Can you work these out from the model? Positions are in its coordinate system, mm. A direction names the side the tool comes from. Give positions to 0.01 mm unless a question says otherwise; leave off trailing zeros. Loops run counter-clockwise (first coordinate to the right, second up) from the corner with the lowest first, then second, coordinate; pieces in that order, holes last. Notation, with made-up numbers: (54, -3) - (93, -3) arc R10 cw to (93, 11) - close; hole circle Ø2 at (76.25, 87). An arc over 180 degrees is marked (long way). Answer as a JSON object with one key per item and string values.
```python
from build123d import *

# Parameters (mm, degrees)
F1_DEPTH = 100
F2_W     = 150
F2_H     = 99.866986
F3_DEPTH = 20
F4_R     = 5
F5_DEPTH = 15


with BuildPart() as f1:
    # F0 (on Top) → F1 (new body)
    with BuildSketch(Plane.XY):
        Polygon((-75, -10), (75, -10), (-75, 10), align=None)
    extrude(amount=F1_DEPTH)

    # F2 (on face) → F3 (join)
    with BuildSketch(Plane.XZ.offset(10)):
        with Locations((0, 49.933493)):
            Rectangle(F2_W, F2_H)
    extrude(amount=F3_DEPTH)

    # F4 (on face) → F5 (join)
    with BuildSketch(Plane(origin=(0, 0, 0), x_dir=(-0.991228, 0.132164, 0), z_dir=(0.132164, 0.991228, 0))):
        with Locations((-68.66373, 45)):
            Circle(F4_R)
    extrude(amount=F5_DEPTH)


solid = f1.part
```
1) I'm going to push a flat-ended pin straight in: P1, Ø2, axis at x = 43.5, y = -21, coming from the +Z side. Where does the tip first touch, or does it pass through?
Check sheet entries:
{"P1": "z = 99.87"}
2) Imagine slicing it at C-C on x = -2.5. Write out the boundary of the cut face in (y, z).
Check sheet entries:
{"outline": "(-30, 0) - (0.33, 0) - (0.33, 100) - (-10, 100) - (-10, 99.87) - (-30, 99.87) - close"}
3) I need wall thicknesses on L1, parallel to Z at x = 1, y = -16.5; L2, parallel to Y at x = 0, z = 16; L3, parallel to Y at x = -7.5, z = 10.5. Which ranges of each line are inside material? Lowest first, please.
Check sheet entries:
{"L1": "0 to 99.87", "L2": "-30 to 0", "L3": "-30 to 1"}
4) Imagine slicing it at A-A on x = -48. Write out the boundary of the cut face in (y, z), and give its area (3 significant figures).
Check sheet entries:
{"outline": "(-30, 0) - (6.4, 0) - (6.4, 100) - (-10, 100) - (-10, 99.87) - (-30, 99.87) - close", "area": "3,640 mm2"}
5) Imagine slicing it at B-B on z = 9.5. Write out the boundary of the cut face in (x, y).
Check sheet entries:
{"outline": "(-75, -30) - (75, -30) - (75, -10) - (-75, 10) - close"}
6) If we mould it in two halves opening along X, with no side actions, what happens to faces 3 (the flat face through (70.113, 5.784, 45.07)), 4 (the flat face through (-75, -10, 49)), 5 (the cylindrical face through (66.374, -1.389, 49.216)), 6 (the flat face through (-1, -30, 51))? For each: released by +X, released by -X, zero draft, split by the parting line, or undercut.
Check sheet entries:
{"face 3": "released by +X", "face 4": "released by -X", "face 5": "undercut", "face 6": "zero draft"}
7) Which directions (+Z, -Z, +X, -X, +Y, -Y) give clear straight access to the entire face, cutting with the end or side of a thin tool? Please do faces 1 (the flat face through (-1, -20, 99.867)), 2 (the flat face through (75, -20, 49)).
Check sheet entries:
{"face 1": "+Z, +X, -X, -Y", "face 2": "+Z, -Z, +X, +Y, -Y"}
